Check sheet for the modelled part. Datum: model origin and axes. Units: mm. Face numbers are marked on the shaded views. A direction names the side the tool comes from. Round coordinates to 2 decimals unless told otherwise and drop trailing zeros. Order: outer loops, then holes, each group sorted by start corner. A loop starts at its lowest first (then second) coordinate and runs counter-clockwise, first axis right, second up. Notation, with made-up numbers: (-4.5, 62.25) -> (5.5, 62.25) arc R32 cw to (5.5, 89.25) -> close; hole circle Ø3 at (71.25, 78.5). An arc over 180 degrees is marked (long way). Answer in a Markdown table with one row per item.
from build123d import *

# Parameters (mm, degrees)
F1_DEPTH = 63.5
F2_DEPTH = 25.4
F3_DEPTH = 7.9375
F5_R     = 6.35


with BuildPart() as f1:
    # F0 (on Front) → F1 (new body, symmetric)
    with BuildSketch(Plane.XZ):
        Polygon((-41.275, -9.525), (41.275, -9.525), (41.275, 9.525), (22.225, 9.525), (-41.275, 9.525), align=None)
    extrude(amount=F1_DEPTH, both=True)

    # F0 (on Front) → F2 (join, symmetric)
    with BuildSketch(Plane.XZ):
        with BuildLine():
            Line((22.225, 9.525), (41.275, 9.525))
            Line((41.275, 9.525), (41.275, 27.0002))
            ThreePointArc((41.275, 27.0002), (45.92468, 38.22552), (57.15, 42.8752))
            Line((57.15, 42.8752), (60.325, 42.8752))
            Line((60.325, 42.8752), (60.325, 61.9252))
            Line((60.325, 61.9252), (57.15, 61.9252))
            ThreePointArc((57.15, 61.9252), (32.454296, 51.695904), (22.225, 27.0002))
            Line((22.225, 27.0002), (22.225, 9.525))
        make_face()
        Polygon((60.325, 66.675), (60.325, 61.9252), (60.325, 42.8752), (85.725, 42.8752), (85.725, 66.675), align=None)
    extrude(amount=F2_DEPTH, both=True)

    # F0 (on Front) → F3 (join, symmetric)
    with BuildSketch(Plane.XZ):
        with BuildLine():
            add(Edge.make_bspline(
                [(-41.275, 9.525), (-40.671952, 35.93922), (22.924198, 62.560864), (57.15, 61.9252)],
                knots=[0, 0, 0, 0, 111.504536, 111.504536, 111.504536, 111.504536], degree=3))
            Line((-41.275, 9.525), (22.225, 9.525))
            Line((22.225, 9.525), (22.225, 27.0002))
            ThreePointArc((22.225, 27.0002), (32.454296, 51.695904), (57.15, 61.9252))
        make_face()
    extrude(amount=F3_DEPTH, both=True)

    # F0 (on Front) → F4 (revolve)
    with BuildSketch(Plane.XZ):
        Polygon((85.725, 66.675), (85.725, 42.8752), (85.725, 38.1), (111.125, 38.1), (111.125, 66.675), align=None)
    revolve(axis=Axis((85.725, 0, 52.3875), (0, 0, 1)))

    # F5
    f5_edges = [f1.edges().sort_by_distance(p)[0] for p in [
        (-41.275, -63.5, 0),
        (41.275, -63.5, 0),
        (41.275, 63.5, 0),
        (-41.275, 63.5, 0),
    ]]
    fillet(f5_edges, radius=F5_R)


solid = f1.part
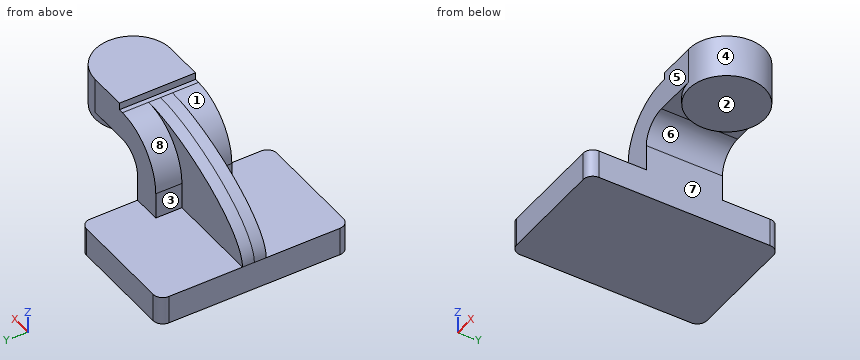
Item 1: Depth check by flat-ended pin: P1, Ø1.4, axis at y = 8, z = 64, coming from the -X side (3 decimals); P2, Ø19, axis at y = -14.5, z = 20, coming from the -X side; P3, Ø6, axis at x = -1, y = 11, coming from the +Z side (3 decimals). Enter the tip coordinate at first touch or a pass-through.
Result sheet:
| item | result |
|---|---|
| P1 | stops at x = 60.325 |
| P2 | stops at x = -40.81 |
| P3 | stops at z = 9.525 |
Item 2: Cross-section at A-A (z = 0.5). Record the boundary of the cut face in (x, y) (3 decimals), and give its area (3 significant figures).
Result sheet:
| item | result |
|---|---|
| outline | (-41.275, -57.15) arc R6.35 ccw to (-34.925, -63.5) -> (34.925, -63.5) arc R6.35 ccw to (41.275, -57.15) -> (41.275, 57.15) arc R6.35 ccw to (34.925, 63.5) -> (-34.925, 63.5) arc R6.35 ccw to (-41.275, 57.15) -> close |
| area | 10,400 mm^2 |
Item 3: Set-up check for the marked faces 1, 2, 3, 4 and 5: record each of +Z, -Z, +X, -X, +Y, -Y from which the full face is reachable in a straight line by a thin tool's end or side.
Result sheet:
| item | result |
|---|---|
| face 1 | +Z, -X, -Y |
| face 2 | -Z, +X, +Y, -Y |
| face 3 | +Z, -X, +Y |
| face 4 | -Z |
| face 5 | +Z, +X, -X, -Y |
Item 4: Mould release check, pull along X, two halves, no side actions. Record for the marked faces 6, 7 and 8: pulls with the +X half, pulls with the -X half, needs draft (parallel to the pull), parting line crosses it, or undercut.
Result sheet:
| item | result |
|---|---|
| face 6 | undercut |
| face 7 | pulls with the +X half |
| face 8 | pulls with the -X half |
Item 5: Cross-section at B-B (x = 67). Record the boundary of the cut face in (y, z) (3 decimals), and give its area (3 significant figures).
Result sheet:
| item | result |
|---|---|
| outline | (-25.4, 42.875) -> (-17.162, 42.875) -> (-17.162, 38.1) -> (17.162, 38.1) -> (17.162, 42.875) -> (25.4, 42.875) -> (25.4, 66.675) -> (-25.4, 66.675) -> close |
| area | 1,370 mm^2 |
Item 6: Scan lines: line 1 (Y direction, x = -21.5, z = 14); line 2 (X direction, y = -51, z = 3) (3 decimals); line 3 (Z direction, x = 56, y = 18.5). Record each from-to range of solid material in increasing order. Write a range as [from, to].
Result sheet:
| item | result |
|---|---|
| line 1 | y = [-7.94, 7.94] |
| line 2 | x = [-41.275, 41.275] |
| line 3 | z = [42.83, 61.91] |
